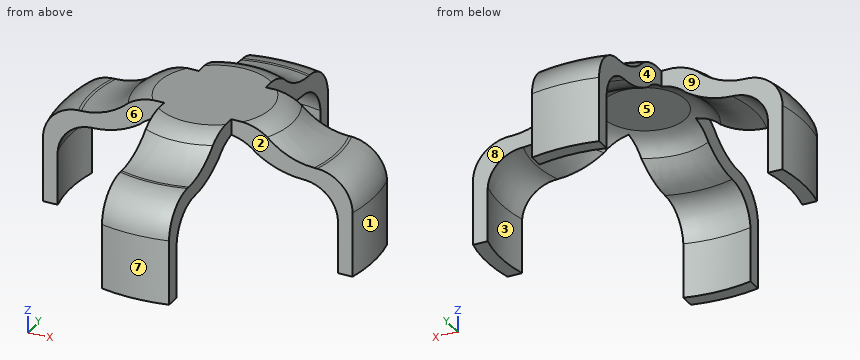
```python
from build123d import *

# Parameters (mm, degrees)
F2_W     = 7.197865
F2_H     = 7.241845
F2_W_2   = 7.277308
F2_H_2   = 7.777737
F2_W_3   = 7.559205
F2_H_3   = 7.282023
F2_W_4   = 6.779674
F2_H_4   = 6.794866
F3_DEPTH = 25.4


with BuildPart() as f1:
    # F0 (on Front) → F1 (revolve)
    with BuildSketch(Plane.XZ):
        with BuildLine():
            Line((2.966464, 6.858), (0, 6.858))
            Line((0, 6.858), (0, 6.096))
            Line((0, 6.096), (2.144658, 6.096))
            ThreePointArc((2.144658, 6.096), (2.920532, 5.876714), (3.557912, 5.382938))
            ThreePointArc((3.557912, 5.382938), (4.622787, 4.797905), (5.8166, 4.572))
            ThreePointArc((5.8166, 4.572), (7.055252, 4.085911), (7.6327, 2.887122))
            Line((7.6327, 2.887122), (7.6327, 0))
            Line((7.6327, 0), (8.3947, 0))
            Line((8.3947, 0), (8.3947, 3.42098))
            ThreePointArc((8.3947, 3.42098), (7.867128, 4.738692), (6.5786, 5.334))
            Line((6.5786, 5.334), (6.428647, 5.334))
            ThreePointArc((6.428647, 5.334), (5.158581, 5.617736), (4.09507, 6.367748))
            ThreePointArc((4.09507, 6.367748), (3.567043, 6.696386), (2.966464, 6.858))
        make_face()
    revolve(axis=Axis((0, 0, 5.133816), (0, 0, 1)))

    # F2 (on Top) → F3 (cut)
    with BuildSketch(Plane.XY):
        with Locations((-5.376932, -5.398923)):
            Rectangle(F2_W, F2_H)
        with Locations((5.416654, -5.666868)):
            Rectangle(F2_W_2, F2_H_2)
        with Locations((5.557602, 5.419011)):
            Rectangle(F2_W_3, F2_H_3)
        with Locations((-5.167837, 5.175433)):
            Rectangle(F2_W_4, F2_H_4)
    extrude(amount=F3_DEPTH, mode=Mode.SUBTRACT)


solid = f1.part
```
Read the model definition and answer for the solid it produces. Units are mm, in the model's axes. Face numbers are marked on the shaded views. A direction names the side the tool comes from. Give positions to 0.01 mm unless a question says otherwise; leave off trailing zeros. Loops run counter-clockwise (first coordinate to the right, second up) from the corner with the lowest first, then second, coordinate; pieces in that order, holes last.
Item 1: For the marked faces 5, 6, 7, 8 and 9, determine the directions among +Z, -Z, +X, -X, +Y, -Y from which every point of the face is accessible in a straight line to the end or side of a thin tool.
Item 2: Each of these flat-tipped pins is pushed along its axis until it touches: pin 1 Ø3 at (x, z) = (-4.5, 4) entering from +Y; pin 2 Ø2 at (x, y) = (3.5, -2.5) entering from -Z; pin 3 Ø3 at (x, z) = (-4.5, 1) entering from +Y; pin 4 Ø2 at (y, z) = (6.5, 5.5) entering from +X. Where does it stop, or does it pass through?
Item 3: The mould has two halves that part along Y. Classify the marked faces 1, 2, 3 and 4: released by +Y, released by -Y, zero draft, split by the parting line, or undercut.
Item 4: The part is cut by section A-A (z = 2). Write down the section's boundary in (x, y).
Item 5: The part is cut by section B-B (z = 3.75). Write down the section's boundary in (x, y), and give its area (3 significant figures).
Item 6: Find the intervals of material crossed by line 1 along Z through (x, y) = (-2, 0); line 2 along X through (y, z) = (4.25, 5.25), in increasing order.
Taken from the geometry:
1. face 5: -Z
1. face 6: +Z, -Z, -X, -Y
1. face 7: +Z, -Z, -Y
1. face 8: +Z, -Z, +X, +Y
1. face 9: +Z, -Z, -X, +Y
2. pin 1: stops at y = 1.78
2. pin 2: stops at z = 4.82
2. pin 3: passes through
2. pin 4: stops at x = 1.78
3. face 1: split by the parting line
3. face 2: released by -Y
3. face 3: undercut
3. face 4: zero draft
4. outline: (-8.2, -1.78) - (-7.42, -1.78) arc R7.63 cw to (-7.42, 1.78) - (-8.2, 1.78) arc R8.39 ccw to start; (-1.78, -8.2) arc R8.39 ccw to (1.78, -8.2) - (1.78, -7.42) arc R7.63 cw to (-1.78, -7.42) - close; (-1.78, 7.42) arc R7.63 cw to (1.78, 7.42) - (1.78, 8.2) arc R8.39 ccw to (-1.78, 8.2) - close; (7.42, -1.78) - (8.2, -1.78) arc R8.39 ccw to (8.2, 1.78) - (7.42, 1.78) arc R7.63 cw to start
5. outline: (-8.17, -1.78) - (-7.12, -1.78) arc R7.34 cw to (-7.12, 1.78) - (-8.17, 1.78) arc R8.37 ccw to start; (-1.78, -8.17) arc R8.37 ccw to (1.78, -8.17) - (1.78, -7.12) arc R7.34 cw to (-1.78, -7.12) - close; (-1.78, 7.12) arc R7.34 cw to (1.78, 7.12) - (1.78, 8.17) arc R8.37 ccw to (-1.78, 8.17) - close; (7.12, -1.78) - (8.17, -1.78) arc R8.37 ccw to (8.17, 1.78) - (7.12, 1.78) arc R7.34 cw to start
5. area: 14.7 mm2
6. line 1: z = 6.1 to 6.86
6. line 2: x = -1.78 to 1.78
